Geometry: see drawing. Coordinates: mm, zero at the bounding-box minimum. A direction names the side the tool comes from. Round coordinates to 2 decimals unless told otherwise and drop trailing zeros. Loops run counter-clockwise (first coordinate to the right, second up) from the corner with the lowest first, then second, coordinate; pieces in that order, holes last. Notation, with made-up numbers: (65, -7) - (86, -7) arc R21 ccw to (86, 0) - close; hole circle Ø5 at (-5, -37.5). An arc over 180 degrees is marked (long way). Use CSV: the item, a comma, the result in double quotes. Start each with the question number.
1. Cut plane A-A (x = 29). Return loops of the section in (y, z).
2. Cut plane C-C (z = 17.75). Return loops of the section in (x, y), and give its area (3 significant figures).
3. Access query for the marked faces 1 and 2. Directions: +Z, -Z, +X, -X, +Y, -Y. A direction counts if a zero-diameter tool reaches every point of the face in a straight line with its end or side. Return the directions, or none.
4. Material intervals for probe 1 along Z at (x, y) = (24, 21.5); probe 2 along Y at (x, z) = (29.5, 16); probe 3 along Z at (x, y) = (33, 33.5), sorted ascending. Write a range as from..to.
5. Pin query (flat end, axial travel): P1, Ø1, axis at x = 43, y = 21, coming from the +Z side; P2, Ø2, axis at x = 51.5, y = 37, coming from the -Z side; P3, Ø2, axis at x = 44.5, z = 7, coming from the +Y side; P4, Ø2, axis at x = 25, z = 16, coming from the -Y side. Return the tip coordinate at first contact, or that it passes through.
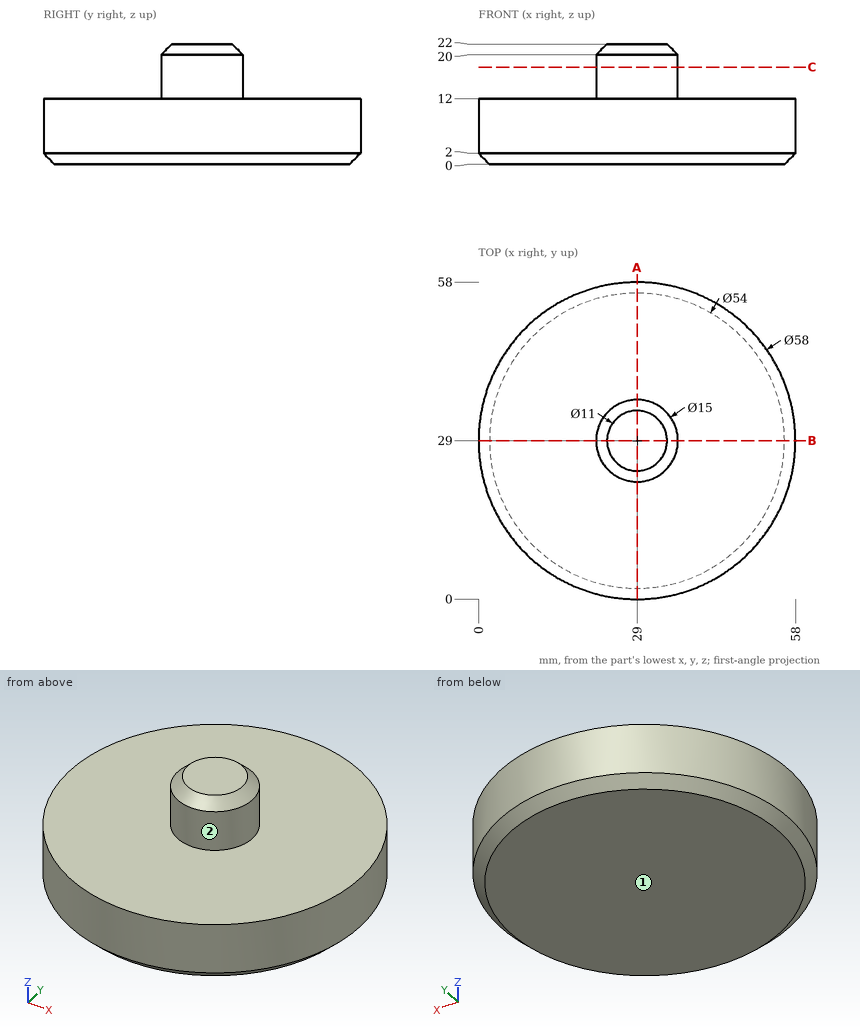
Established:
1,outline,"(0, 2) - (2, 0) - (56, 0) - (58, 2) - (58, 12) - (36.5, 12) - (36.5, 20) - (34.5, 22) - (23.5, 22) - (21.5, 20) - (21.5, 12) - (0, 12) - close"
2,outline,"circle Ø15 at (29, 29)"
2,area,"177 mm2"
3,face 1,"-Z, +X, -X, +Y, -Y"
3,face 2,"+Z"
4,probe 1,"z = 0..12"
4,probe 2,"y = 21.52..36.48"
4,probe 3,"z = 0..21.48"
5,P1,"stops at z = 12"
5,P2,"stops at z = 0"
5,P3,"stops at y = 54.11"
5,P4,"stops at y = 22.13"
